Check sheet for the modelled part. Datum: model origin and axes. Units: mm. A direction names the side the tool comes from. Round coordinates to 2 decimals unless told otherwise and drop trailing zeros. Loops run counter-clockwise (first coordinate to the right, second up) from the corner with the lowest first, then second, coordinate; pieces in that order, holes last. Notation, with made-up numbers: M -26,41.25 L 20,41.25 A35 cw 20,74.25 Z; hole C 66.5,53 d2. An arc over 180 degrees is marked long. Write item = value, one per line. Start each with the question number.
(1) Go/stop test with flat-tipped pins: P1, Ø8, axis at y = 5, z = 10, coming from the -X side; P2, Ø1.9, axis at x = -4, z = 28, coming from the +Y side; P3, Ø0.9, axis at x = 4, z = 34.5, coming from the -Y side. Record where each tip stops, or that it passes through.
(2) Cross-section at C-C on z = 5. Record the boundary of the cut face in (x, y), plus the area to 3 significant figures.
(3) Cross-section at A-A on y = 0. Record the boundary of the cut face in (x, z), plus the area to 3 significant figures.
(4) Cross-section at B-B on x = 0. Record the boundary of the cut face in (y, z).
(5) Cross-section at D-D on y = -3.5. Record the boundary of the cut face in (x, z), plus the area to 3 significant figures.
(6) Set-up check for faces 1 (the face through (2.5, 0.1, 7.1)), 2 (the face through (-2, 0, 0)), 3 (the face through (-4, -1.5, 33)): record each of +Z, -Z, +X, -X, +Y, -Y from which the full face is reachable in a straight line by a thin tool's end or side.
(7) Mould release check, pull along X, two halves, no side actions. Record for faces 4 (the face through (6.466, -2.681, 22.185)), 5 (the face through (3, 0, 33)), 6 (the face through (-3.2, 0.1, 45)): pulls with the +X half, pulls with the -X half, needs draft (parallel to the pull), parting line crosses it, or undercut.
(8) Scan lines: L1, parallel to Y at x = 0, z = 6; L2, parallel to X at y = -2.5, z = 35.5; L3, parallel to X at y = -4.5, z = 27. Record each from-to range of solid material in increasing order. Write a range as from..to.
from build123d import *

# Parameters (mm, degrees)
F0_R     = 7
F1_DEPTH = 45
F3_DEPTH = 25
F4_R     = 2.55
F5_DEPTH = 10
F7_DEPTH = 4
F8_DEPTH = 10


with BuildPart() as f1:
    # F0 (on Top) → F1 (new body)
    with BuildSketch(Plane.XY):
        Circle(F0_R)
    extrude(amount=F1_DEPTH)

    # F2 (on face) → F3 (cut)
    with BuildSketch(Plane.XY.offset(45)):
        with BuildLine():
            ThreePointArc((4.7696960071, 1.5), (0, 5), (-4.7696960071, 1.5))
            Line((-4.7696960071, 1.5), (-3, 1.5))
            Line((-3, 1.5), (-3, -1.5))
            Line((-3, -1.5), (-4.7696960071, -1.5))
            ThreePointArc((-4.7696960071, -1.5), (0, -5), (4.7696960071, -1.5))
            Line((4.7696960071, -1.5), (3, -1.5))
            Line((3, -1.5), (3, 1.5))
            Line((3, 1.5), (4.7696960071, 1.5))
        make_face()
    extrude(amount=-F3_DEPTH, mode=Mode.SUBTRACT)

    # F4 (on face) → F5 (cut)
    with BuildSketch(Plane(origin=(0, 0, 0), x_dir=(1, 0, 0), z_dir=(0, 0, -1))):
        Circle(F4_R)
    extrude(amount=-F5_DEPTH, mode=Mode.SUBTRACT)

    # F6 (on face) → F7 (cut)
    with BuildSketch(Plane(origin=(0, 0, 10), x_dir=(1, 0, 0), z_dir=(0, 0, -1))):
        with BuildLine():
            Line((-1.5, 2), (-1.5, -2))
            ThreePointArc((-1.5, -2), (2.5, 0), (-1.5, 2))
        make_face()
    extrude(amount=-F7_DEPTH, mode=Mode.SUBTRACT)

    # F8 (add): a face of the model
    f8_faces = [f1.faces().sort_by_distance(p)[0] for p in [
        (-2.4778751083, 0, 10),
    ]]
    extrude(f8_faces, amount=F8_DEPTH)


solid = f1.part
Result:
q1.P1 = -6.93
q1.P2 = 6.3
q1.P3 = -6.03
q2.outline = C 0,0 d14; hole M -1.5,-2 A2.5 ccw long -1.5,2 Z
q2.area = 137 mm^2
q3.outline = M -7,0 L -1.5,0 L -1.5,14 L 2.5,14 L 2.5,0 L 7,0 L 7,45 L 3,45 L 3,20 L -3,20 L -3,45 L -7,45 Z
q3.area = 424 mm^2
q4.outline = M -7,0 L -2.5,0 L -2.5,14 L 2.5,14 L 2.5,0 L 7,0 L 7,45 L 5,45 L 5,20 L -5,20 L -5,45 L -7,45 Z
q5.outline = M -6.06,0 L 6.06,0 L 6.06,45 L 3.57,45 L 3.57,20 L -3.57,20 L -3.57,45 L -6.06,45 Z
q5.area = 367 mm^2
q6.face_1 = -Z
q6.face_2 = -Z, +X, -X, +Y, -Y
q6.face_3 = +Z
q7.face_4 = parting line crosses it
q7.face_5 = undercut
q7.face_6 = needs draft
q8.L1 = -7..-2.5, 2.5..7
q8.L2 = -6.54..-4.33, 4.33..6.54
q8.L3 = -5.36..-2.18, 2.18..5.36
